```python
from build123d import *

# Parameters (mm, degrees)
CHAMFER6_SIZE   = 4
CHAMFER6_SIZE_2 = 6.92820323
CHAMFER4_SIZE   = 2


with BuildPart() as part:
    # Sketch3 → Revolve2 (revolve)
    with BuildSketch(Plane.XY, mode=Mode.PRIVATE) as revolve2_sk:
        Polygon((8, 6), (8, 10), (4, 10), (4, 6), (4, 3), (7, 3), (7, 1), (7, -1), (10, -1), (10, 6), align=None)
    revolve(revolve2_sk.sketch.rotate(Axis((0, 50.624065585, 0), (0, -1, 0)), 90), axis=Axis((0, 50.624065585, 0), (0, -1, 0)))

    # Chamfer6
    # the kernel refuses this chamfer: 6.92820323, 4 mm, written as the material it takes off along each edge
    with BuildSketch(Plane(origin=(0, 10, 0), x_dir=(0, 0, 1), z_dir=(1, 0, 0))) as chamfer6_piece_1_section:
        Polygon((8, CHAMFER6_SIZE), (8 - CHAMFER6_SIZE_2, 0), (8, 0), align=None)
    chamfer6_piece_1 = revolve(axis=Axis((0, 10, 0), (0, -1, 0)), mode=Mode.PRIVATE)
    chamfer6_piece_1 = split(chamfer6_piece_1, bisect_by=Plane(origin=(0, 6, -4.457093256), z_dir=(0, 1, 0)), keep=Keep.TOP, mode=Mode.PRIVATE)
    add(chamfer6_piece_1, mode=Mode.SUBTRACT)

    # Chamfer4
    chamfer4_edges = [part.edges().sort_by_distance(p)[0] for p in [
        (0, -1, -7),
    ]]
    chamfer(chamfer4_edges, length=CHAMFER4_SIZE)


solid = part.part
```
Geometry: final body of the model. Coordinates: model frame, mm. Coordinates: 2 decimals unless noted, no trailing zeros. Loops run counter-clockwise (first coordinate to the right, second up) from the corner with the lowest first, then second, coordinate; pieces in that order, holes last. Notation, with made-up numbers: (5, 31.25) -> (17, 31.25) arc R19 cw to (17, 66.25) -> close; hole circle Ø10 at (68.25, 26). An arc over 180 degrees is marked (long way). Use a Markdown table: item, result. Add a question column.
(1) Section query C-C, the plane y = 4. Return loops of the section in (x, z).
(2) Mould query, pull axis Z, two halves, no side actions, for faces 1 (the cylindrical face through (0, 3, -10)), 2 (the cylindrical face through (6.21, 1.99, 3.23)), 3 (the flat face through (-8.2, 6, 0)), 4 (the flat face through (3, 3, -3)). Classes: pulls with the +Z half, pulls with the -Z half, needs draft (parallel to the pull), parting line crosses it, or undercut.
(3) Pin query (flat end, axial travel): pin 1 Ø1 at (y, z) = (4, 3) entering from -X; pin 2 Ø2 at (x, z) = (-6.5, -7) entering from +Y; pin 3 Ø1 at (x, y) = (7, 2) entering from +Z; pin 4 Ø4 at (x, z) = (-1, 0) entering from -Y. Return the tip coordinate at first contact, or that it passes through.
(4) Section query A-A, the plane x = 0. Return loops of the section in (y, z).
(5) Line query: line 1 along X through (y, z) = (4.4, 0); line 2 along Y through (x, z) = (-9, 0.5); line 3 along X through (y, z) = (2.5, 1.75). Output: solid intervals per line, ascending.
(6) Section query D-D, the plane y = 2. Return loops of the section in (x, z), plus the area to 3 significant figures.
(7) Section query B-B, the plane z = 0. Return loops of the section in (x, y).
Answer:
| question | item | result |
|---|---|---|
| 1 | outline | circle Ø20 at (0, 0); hole circle Ø8 at (0, 0) |
| 2 | face 1 | parting line crosses it |
| 2 | face 2 | undercut |
| 2 | face 3 | needs draft |
| 2 | face 4 | undercut |
| 3 | pin 1 | stops at x = -9.68 |
| 3 | pin 2 | stops at y = 6 |
| 3 | pin 3 | stops at z = 7.6 |
| 3 | pin 4 | passes through |
| 4 | outline | (-1, -10) -> (6, -10) -> (6, -8) -> (8.31, -4) -> (3, -4) -> (3, -7) -> (1, -7) -> (-1, -9) -> close; (-1, 9) -> (1, 7) -> (3, 7) -> (3, 4) -> (8.31, 4) -> (6, 8) -> (6, 10) -> (-1, 10) -> close |
| 5 | line 1 | x = -10 to -4, 4 to 10 |
| 5 | line 2 | y = -1 to 6 |
| 5 | line 3 | x = -9.85 to -6.78, 6.78 to 9.85 |
| 6 | outline | circle Ø20 at (0, 0); hole circle Ø14 at (0, 0) |
| 6 | area | 160 mm^2 |
| 7 | outline | (-10, -1) -> (-9, -1) -> (-7, 1) -> (-7, 3) -> (-4, 3) -> (-4, 8.31) -> (-8, 6) -> (-10, 6) -> close; (4, 3) -> (7, 3) -> (7, 1) -> (9, -1) -> (10, -1) -> (10, 6) -> (8, 6) -> (4, 8.31) -> close |
